Design review of the part built by this model. Coordinates are the model's own, in mm. Face numbers are marked on the shaded views. Give positions to 0.01 mm unless a question says otherwise; leave off trailing zeros. Write each loop counter-clockwise with the first axis right and the second up, starting at its lowest first coordinate (ties: lowest second). Pieces come first, ordered by that corner, then holes. Notation, with made-up numbers: M -32,52 L 16,52 A17 ccw 16,66 Z; hole C -13,27 d7. An arc over 180 degrees is marked long. Answer in a Markdown table with one row per item.
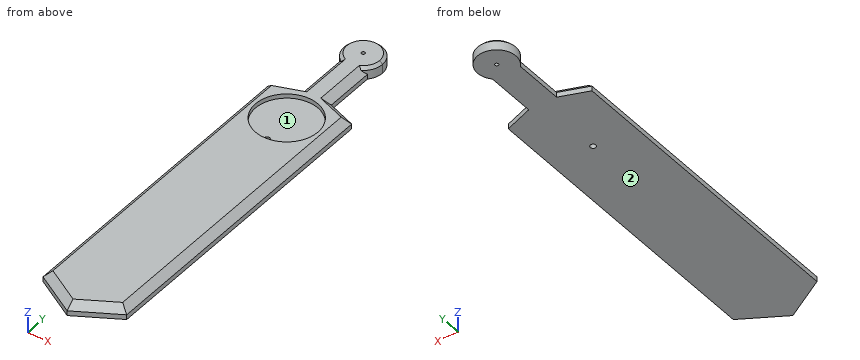
```python
from build123d import *

# Parameters (mm, degrees)
F1_DEPTH = 21.59
F2_R     = 56.896
F3_DEPTH = 7.874
F4_R     = 5.08
F5_DEPTH = 13.717
F6_SIZE  = 12.7
F7_R     = 3.175
F8_DEPTH = 21.591
F9_SIZE  = 5.08


with BuildPart() as f1:
    # F0 (on Top) → F1 (new body)
    with BuildSketch(Plane.XY):
        with BuildLine():
            Line((25.4, -23.970724332), (25.4, 0))
            ThreePointArc((25.4, 0), (0, -25.4), (-25.4, 0))
            Line((-25.4, 0), (-25.4, -23.970724332))
            ThreePointArc((-25.4, -23.970724332), (0, -34.925), (25.4, -23.970724332))
        make_face()
        with BuildLine():
            Line((25.4, -114.3), (25.4, -23.970724332))
            ThreePointArc((25.4, -23.970724332), (0, -34.925), (-25.4, -23.970724332))
            Line((-25.4, -23.970724332), (-25.4, -114.3))
            Line((-25.4, -114.3), (-76.2, -132.7896879007))
            Line((-76.2, -132.7896879007), (-76.2, -692.6059094878))
            Line((-76.2, -692.6059094878), (0, -736.6))
            Line((0, -736.6), (76.2, -692.6059094878))
            Line((76.2, -692.6059094878), (76.2, -132.7896879007))
            Line((76.2, -132.7896879007), (25.4, -114.3))
        make_face()
        with BuildLine():
            ThreePointArc((-25.4, 0), (0, -25.4), (25.4, 0))
            ThreePointArc((25.4, 0), (0, 25.4), (-25.4, 0))
        make_face()
        with BuildLine():
            ThreePointArc((-25.4, 0), (0, 25.4), (25.4, 0))
            Line((25.4, 0), (25.4, -23.970724332))
            ThreePointArc((25.4, -23.970724332), (32.4565141767, -12.8969109674), (34.925, 0))
            ThreePointArc((34.925, 0), (-12.8969109674, 32.4565141767), (-25.4, -23.970724332))
            Line((-25.4, -23.970724332), (-25.4, 0))
        make_face()
    extrude(amount=F1_DEPTH)

    # F2 (on face) → F3 (cut)
    with BuildSketch(Plane.XY.offset(21.59)):
        with Locations((0, -190.5)):
            Circle(F2_R)
    extrude(amount=-F3_DEPTH, mode=Mode.SUBTRACT)

    # F4 (on face) → F5 (cut, through all)
    with BuildSketch(Plane.XY.offset(13.716)):
        with Locations((0, -239.776)):
            Circle(F4_R)
    extrude(amount=-F5_DEPTH, mode=Mode.SUBTRACT)

    # F6
    f6_edges = [f1.edges().sort_by_distance(p)[0] for p in [
        (-76.2, -412.697799, 21.59),
        (-38.1, -714.602955, 21.59),
        (38.1, -714.602955, 21.59),
        (76.2, -412.697799, 21.59),
        (50.8, -123.544844, 21.59),
        (-50.8, -123.544844, 21.59),
        (25.4, -69.135362, 21.59),
        (-25.4, -69.135362, 21.59),
    ]]
    chamfer(f6_edges, length=F6_SIZE)

    # F7 (on face) → F8 (cut, through all)
    with BuildSketch(Plane.XY.offset(21.59)):
        Circle(F7_R)
    extrude(amount=-F8_DEPTH, mode=Mode.SUBTRACT)

    # F9
    f9_edges = [f1.edges().sort_by_distance(p)[0] for p in [
        (0, 34.925, 21.59),
    ]]
    chamfer(f9_edges, length=F9_SIZE)


solid = f1.part
```
1) To check wall thickness, follow probe 1 along Y at (x, z) = (0, 5) (3 decimals); probe 2 along Y at (x, z) = (0, 17.25) (3 decimals); probe 3 along X at (y, z) = (-208, 19.75). State the ranges of each line that lie inside material, in increasing order. Write a range as [from, to].
Geometry says:
| item | result |
|---|---|
| probe 1 | [-736.6, -244.856], [-234.696, -3.175], [3.175, 34.925] |
| probe 2 | [-726.947, -247.396], [-133.604, -3.175], [3.175, 34.185] |
| probe 3 | [-65.34, -54.14], [54.14, 65.34] |
2) Add section A-A (y = -190.5). Write out the cut boundary in (x, z), and give its area (3 significant figures).
Geometry says:
| item | result |
|---|---|
| outline | M -76.2,0 L 76.2,0 L 76.2,8.89 L 63.5,21.59 L 56.9,21.59 L 56.9,13.72 L -56.9,13.72 L -56.9,21.59 L -63.5,21.59 L -76.2,8.89 Z |
| area | 2,230 mm^2 |
3) Add section B-B (y = -400). Write out the cut boundary in (x, z).
Geometry says:
| item | result |
|---|---|
| outline | M -76.2,0 L 76.2,0 L 76.2,8.89 L 63.5,21.59 L -63.5,21.59 L -76.2,8.89 Z |
4) Insertion check: P1, Ø6, axis at x = 19, z = 6.5, coming from the -Y side; P2, Ø2.5, axis at y = -88.5, z = 6, coming from the +X side; P3, Ø6, axis at x = 54, z = 5.5, coming from the -Y side. Each pin has a flat end and moves straight along its axis. Give the tip position at first contact, or say it passes through.
Geometry says:
| item | result |
|---|---|
| P1 | y = -727.36 |
| P2 | x = 25.4 |
| P3 | y = -707.16 |
5) The part is to be moulded in two halves that separate along X. For the marked faces 1 and 2, say which applies: released by +X, released by -X, zero draft, split by the parting line, or undercut.
Geometry says:
| item | result |
|---|---|
| face 1 | undercut |
| face 2 | zero draft |
